Could you check a few things on this drawing? It's one solid part, dimensions in mm from its lowest x, y, z. A direction names the side the tool comes from. Give positions to 0.01 mm unless a question says otherwise; leave off trailing zeros. Order: outer loops, then holes, each group sorted by start corner. A loop starts at its lowest first (then second) coordinate and runs counter-clockwise, first axis right, second up. Notation, with made-up numbers: M 63.25,81.25 L 112.25,81.25 A21 ccw 112.25,106.25 Z; hole C 63.25,-1 d7. An arc over 180 degrees is marked long. Use one line per item in the form item = value. Start each with the question number.
1. I want a section at A-A, the plane x = 35. List the corners of the cut face in (y, z) for me.
2. For the marked faces 1 and 2, which set-ups out of +Z, -Z, +X, -X, +Y, -Y let a thin tool reach every point of the face, with its end or its side?
3. I want a section at B-B, the plane z = 4. List the corners of the cut face in (x, y) for me.
4. I want a section at C-C, the plane x = 15. List the corners of the cut face in (y, z) for me.
5. I need wall thicknesses on L1, parallel to Z at x = 3, y = 1.2; L2, parallel to X at y = 2.7, z = 4; L3, parallel to X at y = 1.25, z = 26. Which ranges of each line are inside material? Lowest first, please.
6. I want a section at D-D, the plane y = 3.3. List the corners of the cut face in (x, z) for me (1 decimal), and give its area (3 significant figures).
7. Will these pins go through, and if not, where does the flat tip stop? P1, Ø1.5, axis at x = 29.5, z = 10, coming from the -Y side; P2, Ø1.8, axis at x = 27, z = 4, coming from the -Y side; P3, Ø1, axis at y = 3, z = 12.5, coming from the -X side (1 decimal).
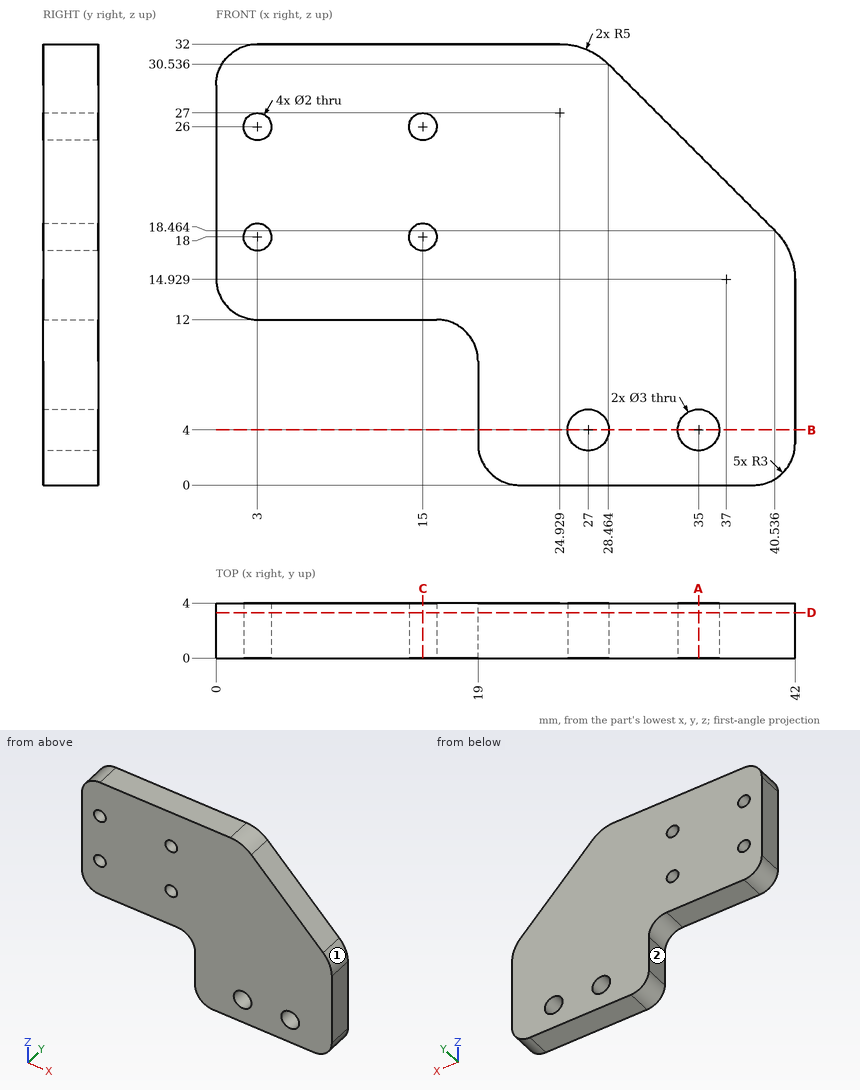
Check result:
q1.outline = M 0,0 L 4,0 L 4,2.5 L 0,2.5 Z; M 0,5.5 L 4,5.5 L 4,24 L 0,24 Z
q2.face_1 = +Z, +X, +Y, -Y
q2.face_2 = -Z, -X, +Y, -Y
q3.outline = M 19,0 L 25.5,0 L 25.5,4 L 19,4 Z; M 28.5,0 L 33.5,0 L 33.5,4 L 28.5,4 Z; M 36.5,0 L 42,0 L 42,4 L 36.5,4 Z
q4.outline = M 0,12 L 4,12 L 4,17 L 0,17 Z; M 0,19 L 4,19 L 4,25 L 0,25 Z; M 0,27 L 4,27 L 4,32 L 0,32 Z
q5.L1 = 12 to 17, 19 to 25, 27 to 32
q5.L2 = 19 to 25.5, 28.5 to 33.5, 36.5 to 42
q5.L3 = 0 to 2, 4 to 14, 16 to 33
q6.outline = M 0,15 A3 ccw 3,12 L 16,12 A3 cw 19,9 L 19,3 A3 ccw 22,0 L 39,0 A3 ccw 42,3 L 42,14.9 A5 ccw 40.5,18.5 L 28.5,30.5 A5 ccw 24.9,32 L 3,32 A3 ccw 0,29 Z; hole C 3,18 d2; hole C 3,26 d2; hole C 15,18 d2; hole C 15,26 d2; hole C 27,4 d3; hole C 35,4 d3
q6.area = 970 mm2
q7.P1 = 0
q7.P2 = through
q7.P3 = 0.8
